The model under review builds one solid part; all positions refer to its coordinate system, in mm. Face numbers are marked on the shaded views. A direction names the side the tool comes from. Coordinates: 2 decimals unless noted, no trailing zeros. Write each loop counter-clockwise with the first axis right and the second up, starting at its lowest first coordinate (ties: lowest second). Pieces come first, ordered by that corner, then holes. Notation, with made-up numbers: (-27.5, 26) - (8.5, 26) arc R14 ccw to (8.5, 46) - close; hole circle Ø4 at (53, -36). An arc over 180 degrees is marked (long way). Put each result on its own line as item: value. Start each with the question number.
Item 1: For pin 1 (1.9 mm diameter, centred on x = 14, z = 1, fed in from +Y); pin 2 (1.1 mm diameter, centred on y = 51, z = 1.5, fed in from +X); pin 3 (3 mm diameter, centred on x = -16, y = 47.5, fed in from -Z); pin 4 (1.2 mm diameter, centred on y = 52.5, z = 1.5, fed in from -X), all flat-tipped, find the tip position at first contact; note any pin that passes through.
Item 2: Consider section B-B on x = -24. Give the boundary of the cut face in (y, z).
Item 3: Mouldability with a two-part tool opening along Y and no side actions: class the marked faces 1, 2, 3 and 4 as pulls with the +Y half, pulls with the -Y half, needs draft (parallel to the pull), parting line crosses it, or undercut.
Item 4: Consider section C-C on y = 52. Give the boundary of the cut face in (x, z).
Item 5: Consider section A-A on x = 3.5. Give the boundary of the cut face in (y, z), then the cut area to 3 significant figures.
Item 6: To check wall thickness, follow L1, parallel to Y at x = -27, z = 2.35; L2, parallel to Y at x = -29, z = 2.9; L3, parallel to X at y = 55, z = 1.65. State the ranges of each line that lie inside material, in increasing order. Write a range as [from, to].
Item 7: Machinability: for the marked faces 5 and 6, which of the approach directions +Z, -Z, +X, -X, +Y, -Y give a long, thin tool a straight path to every point of the face, cutting with its end or side? Answer none if there is none.
Item 8: Consider section D-D on x = -18.5. Give the boundary of the cut face in (y, z).
```python
from build123d import *

# Parameters (mm, degrees)
EXTRUDE_1_DEPTH = 4
FILLET_1_R      = 1.3


with BuildPart() as part:
    # 草图1 → 凸台-拉伸1 (new body)
    with BuildSketch(Plane.XY):
        Polygon((-33.523824953, 29.589854129), (-28.523824953, 29.589854129), (11.476175047, 29.589854129), (16.476175047, 29.589854129), (16.476175047, 37.589854129), (11.476175047, 37.589854129), (11.476175047, 47.089854129), (8.976175047, 47.089854129), (8.976175047, 45.739854129), (6.276175047, 45.739854129), (6.276175047, 47.089854129), (2.076175047, 47.089854129), (2.076175047, 50.089854129), (6.276175047, 50.089854129), (6.276175047, 51.439854129), (8.976175047, 51.439854129), (8.976175047, 50.089854129), (11.476175047, 50.089854129), (11.476175047, 59.589854129), (-24.523824953, 67.589854129), (-28.523824953, 67.589854129), (-33.523824953, 67.589854129), (-33.523824953, 59.589854129), (-28.523824953, 59.589854129), (-28.523824953, 50.089854129), (-26.023824953, 50.089854129), (-26.023824953, 51.439854129), (-23.323824953, 51.439854129), (-23.323824953, 50.089854129), (-19.123824953, 50.089854129), (-19.123824953, 47.089854129), (-23.323824953, 47.089854129), (-23.323824953, 45.739854129), (-26.023824953, 45.739854129), (-26.023824953, 47.089854129), (-28.523824953, 47.089854129), (-28.523824953, 37.589854129), (-33.523824953, 37.589854129), align=None)
    extrude(amount=EXTRUDE_1_DEPTH)

    # 圆角1
    fillet_1_edges = [part.edges().sort_by_distance(p)[0] for p in [
        (-33.523824953, 59.589854129, 2),
        (-33.523824953, 67.589854129, 2),
        (16.476175047, 37.589854129, 2),
        (16.476175047, 29.589854129, 2),
        (-33.523824953, 29.589854129, 2),
        (-33.523824953, 37.589854129, 2),
    ]]
    fillet(fillet_1_edges, radius=FILLET_1_R)


solid = part.part
```
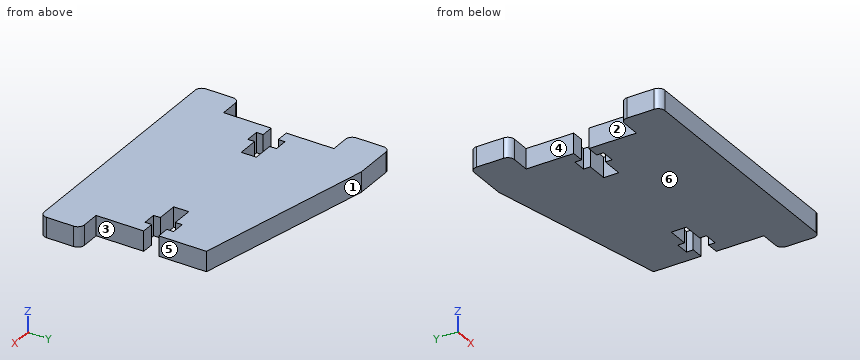
Report:
1. pin 1: y = 37.59
1. pin 2: x = 11.48
1. pin 3: z = 0
1. pin 4: x = -28.52
2. outline: (29.59, 0) - (45.74, 0) - (45.74, 4) - (29.59, 4) - close; (51.44, 0) - (67.47, 0) - (67.47, 4) - (51.44, 4) - close
3. face 1: pulls with the +Y half
3. face 2: undercut
3. face 3: needs draft
3. face 4: undercut
4. outline: (-28.52, 0) - (11.48, 0) - (11.48, 4) - (-28.52, 4) - close
5. outline: (29.59, 0) - (47.09, 0) - (47.09, 4) - (29.59, 4) - close; (50.09, 0) - (61.36, 0) - (61.36, 4) - (50.09, 4) - close
5. area: 115 mm²
6. L1: [29.59, 47.09], [50.09, 67.59]
6. L2: [29.59, 37.59], [59.59, 67.59]
6. L3: [-28.52, 11.48]
7. face 5: +Z, -Z, +X, +Y
7. face 6: -Z, +X, -X, +Y, -Y
8. outline: (29.59, 0) - (66.25, 0) - (66.25, 4) - (29.59, 4) - close
